Here's how the part is built. I have some questions about the finished solid (model axes, mm). Round coordinates to 2 decimals unless told otherwise and drop trailing zeros. Loops run counter-clockwise (first coordinate to the right, second up) from the corner with the lowest first, then second, coordinate; pieces in that order, holes last. Notation, with made-up numbers: (67.5, -0.75) - (76.5, -0.75) arc R17 ccw to (76.5, 31.25) - close; hole circle Ø11 at (68.5, -4.75). An arc over 180 degrees is marked (long way). Return JSON: item names as keys, results as strings. Group by question number.
Solid Edge part; units mm, degrees
sketch "Sketch1" plane through (0, 0, 0) normal (1, 0, 0) x (0, 1, 0)
  circle A0 centre (0, 0) radius 2
extrude "Protrusion1" add sketch "Sketch1" along normal mid plane 84
cosmetic_thread "Thread_1" thread depth 8
cosmetic_thread "Thread_2" thread depth 8
chamfer "Chamfer_1" distance 0.5 angle 45 1 edges at (-42, -2, 0) measured on face at (-42, 1.2933, -1.3733)
chamfer "Chamfer_2" distance 0.5 angle 45 1 edges at (42, -2, 0) measured on face at (42, 1.2933, -1.3733)
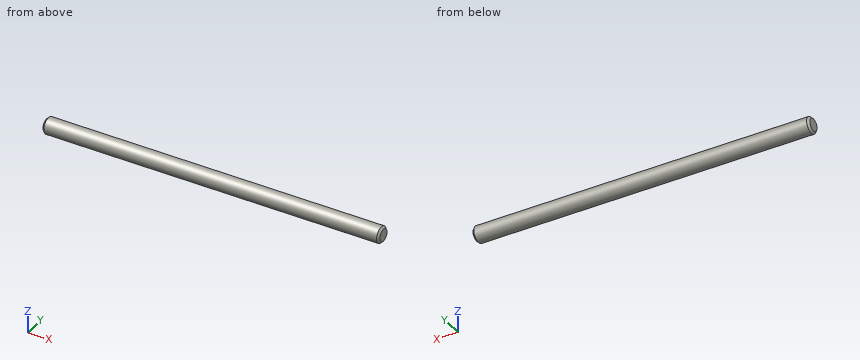
Q1. Imagine slicing it at A-A, the plane x = -6.5. List the corners of the cut face in (y, z) for me, and give its area (3 significant figures).
Q2. Will this pin go through, and if not, where does the flat tip stop? pin 1 Ø2 at (x, y) = (22.5, -1.5) entering from +Z.
Q3. Please list where these lines run through material, in increasing order: line 1 (Z direction, x = 1.5, y = -0.1); line 2 (Y direction, x = 11, z = 1.2); line 3 (Z direction, x = 34, y = -0.65).
Output values:
{
 "1": {"outline": "circle Ø4 at (0, 0)", "area": "12.6 mm^2"},
 "2": {"pin 1": "stops at z = 1.94"},
 "3": {"line 1": "z = -2 to 2", "line 2": "y = -1.6 to 1.6", "line 3": "z = -1.89 to 1.89"}
}
